Source: CAD feature listing. Evaluate the final solid. Frame: model axes, mm. Face numbers are marked on the shaded views. A direction names the side the tool comes from. Give positions to 0.01 mm unless a question says otherwise; leave off trailing zeros. Loops run counter-clockwise (first coordinate to the right, second up) from the corner with the lowest first, then second, coordinate; pieces in that order, holes last.
from build123d import *

# Parameters (mm, degrees)
SKETCH1_W                   = 82
SKETCH1_H                   = 42.5
SKETCH1_W_2                 = 80
SKETCH1_H_2                 = 40.5
VYSUNOUT_TENKOST_NN_1_DEPTH = 10
SKICA1_W                    = 82
SKICA1_H                    = 42.5
P_IDAT_VYSUNUT_M1_DEPTH     = 3
SKETCH3_R                   = 2.2
CUT_EXTRUDE2_DEPTH          = 11
CUT_EXTRUDE2_DEPTH_BACK     = 4


with BuildPart() as part:
    # Sketch1 → Vysunout tenkostěnný1 (new body)
    with BuildSketch(Plane.XY):
        Rectangle(SKETCH1_W, SKETCH1_H)
        Rectangle(SKETCH1_W_2, SKETCH1_H_2, mode=Mode.SUBTRACT)
    extrude(amount=VYSUNOUT_TENKOST_NN_1_DEPTH)

    # Skica1 → Přidat vysunutím1 (add)
    with BuildSketch(Plane.XY):
        Rectangle(SKICA1_W, SKICA1_H)
    extrude(amount=-P_IDAT_VYSUNUT_M1_DEPTH)

    # Sketch3 → Cut-Extrude2 (cut, two sides)
    with BuildSketch(Plane.XY) as cut_extrude2_sk:
        with Locations((0, -17.6)):
            Circle(SKETCH3_R)
        with Locations((0, 17.6)):
            Circle(SKETCH3_R)
    extrude(amount=CUT_EXTRUDE2_DEPTH, mode=Mode.SUBTRACT)
    extrude(cut_extrude2_sk.sketch, amount=-CUT_EXTRUDE2_DEPTH_BACK, mode=Mode.SUBTRACT)


solid = part.part
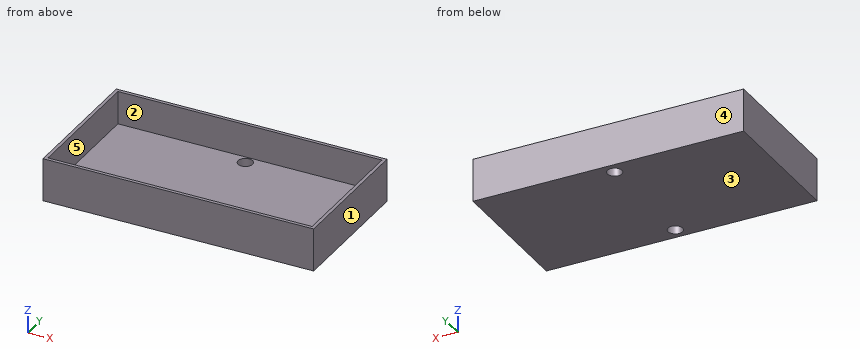
1) Cut plane B-B (z = 4.5). Return loops of the section in (x, y).
Checks:
outline: (-41, -21.25) - (41, -21.25) - (41, 21.25) - (-41, 21.25) - close; hole (-40, -20.25) - (40, -20.25) - (40, 20.25) - (-40, 20.25) - close
2) Ray query, probe 1 along Y at (x, z) = (0, -1.1); probe 2 along X at (y, z) = (10, 9.75); probe 3 along Y at (x, z) = (0, 1.5). Return the intervals inside material, ascending.
Checks:
probe 1: y = -21.25 to -19.8, -15.4 to 15.4, 19.8 to 21.25
probe 2: x = -41 to -40, 40 to 41
probe 3: y = -21.25 to -20.25, 20.25 to 21.25
3) Cut plane C-C (x = 0). Return loops of the section in (y, z), and give its area (3 significant figures).
Checks:
outline: (-21.25, -3) - (-19.8, -3) - (-19.8, 0) - (-20.25, 0) - (-20.25, 10) - (-21.25, 10) - close; (-15.4, -3) - (15.4, -3) - (15.4, 0) - (-15.4, 0) - close; (19.8, -3) - (21.25, -3) - (21.25, 10) - (20.25, 10) - (20.25, 0) - (19.8, 0) - close
area: 121 mm2
4) Pull-direction query (Y, two-part tool) for the marked faces 3, 4 and 5; classes: released by +Y, released by -Y, zero draft, split by the parting line, or undercut.
Checks:
face 3: zero draft
face 4: released by +Y
face 5: undercut
5) Cut plane D-D (y = -5). Return loops of the section in (x, z), and give its area (3 significant figures).
Checks:
outline: (-41, -3) - (41, -3) - (41, 10) - (40, 10) - (40, 0) - (-40, 0) - (-40, 10) - (-41, 10) - close
area: 266 mm2
6) Cut plane A-A (y = 17.6). Return loops of the section in (x, z), and give its area (3 significant figures).
Checks:
outline: (-41, -3) - (-2.2, -3) - (-2.2, 0) - (-40, 0) - (-40, 10) - (-41, 10) - close; (2.2, -3) - (41, -3) - (41, 10) - (40, 10) - (40, 0) - (2.2, 0) - close
area: 253 mm2
7) Contact query for flat-ended pins moving along their axis: P1, Ø20, axis at x = -5, y = -1.5, coming from the +Z side; P2, Ø5.5, axis at x = 0, y = -17.6, coming from the -Z side. Output: stop coordinate, or through.
Checks:
P1: stops at z = 0
P2: stops at z = -3
8) Reachability of the marked faces 1 and 2 from +Z, -Z, +X, -X, +Y, -Y: full face, straight path, thin tool, end or side. Return the list, or none.
Checks:
face 1: +Z, -Z, +X, +Y, -Y
face 2: +Z
